from build123d import *

# Parameters (mm, degrees)
SKETCH1_R                                = 5
BOSS_EXTRUDE2_DEPTH                      = 115.57
CUT_EXTRUDE1_DEPTH                       = 2.54
TAP_DRILL_FOR_10_32_TAP1_D               = 4.0386
TAP_DRILL_FOR_10_32_TAP1_DEPTH           = 11.486682152
TAP_DRILL_FOR_10_32_TAP1_TIP             = 1.213317848
TAP_DRILL_FOR_10_32_TAP1_ON_FACE_2_D     = 4.0386
TAP_DRILL_FOR_10_32_TAP1_ON_FACE_2_DEPTH = 11.486682152
TAP_DRILL_FOR_10_32_TAP1_ON_FACE_2_TIP   = 1.213317848


with BuildPart() as part:
    # Sketch1 → Boss-Extrude2 (new body)
    with BuildSketch(Plane(origin=(0, 0, 0), x_dir=(1, 0, 0), z_dir=(0, 1, 0))):
        Circle(SKETCH1_R)
    extrude(amount=-BOSS_EXTRUDE2_DEPTH)

    # Sketch2 → Cut-Extrude1 (cut)
    with BuildSketch(Plane(origin=(0, 0, -5), x_dir=(-1, 0, 0), z_dir=(0, 0, -1))):
        with BuildLine():
            Line((-2, -109.22), (-2, -114.22))
            ThreePointArc((-2, -114.22), (0, -116.22), (2, -114.22))
            Line((2, -114.22), (2, -109.22))
            ThreePointArc((2, -109.22), (0, -107.22), (-2, -109.22))
        make_face()
        with BuildLine():
            Line((-1.5, -63.5), (-1.5, -68.5))
            ThreePointArc((-1.5, -68.5), (0, -70), (1.5, -68.5))
            Line((1.5, -68.5), (1.5, -63.5))
            ThreePointArc((1.5, -63.5), (0, -62), (-1.5, -63.5))
        make_face()
        with BuildLine():
            Line((-1.5, -10.39), (-1.5, -15.39))
            ThreePointArc((-1.5, -15.39), (0, -16.89), (1.5, -15.39))
            Line((1.5, -15.39), (1.5, -10.39))
            ThreePointArc((1.5, -10.39), (0, -8.89), (-1.5, -10.39))
        make_face()
    extrude(amount=-CUT_EXTRUDE1_DEPTH, mode=Mode.SUBTRACT)

    # Tap Drill for #10-32 Tap1
    with Locations(Plane.ZX):
        with Locations((0, 0)):
            Hole(TAP_DRILL_FOR_10_32_TAP1_D / 2, depth=TAP_DRILL_FOR_10_32_TAP1_DEPTH)
            with Locations((0, 0, -(TAP_DRILL_FOR_10_32_TAP1_DEPTH + TAP_DRILL_FOR_10_32_TAP1_TIP / 2))):  # 118° drill point
                Cone(0, TAP_DRILL_FOR_10_32_TAP1_D / 2, TAP_DRILL_FOR_10_32_TAP1_TIP, mode=Mode.SUBTRACT)

    # Tap Drill for #10-32 Tap1 on face 2
    with Locations(Plane(origin=(0, -115.57, 0), x_dir=(0, 0, -1), z_dir=(0, -1, 0))):
        with Locations((0, 0)):
            Hole(TAP_DRILL_FOR_10_32_TAP1_ON_FACE_2_D / 2, depth=TAP_DRILL_FOR_10_32_TAP1_ON_FACE_2_DEPTH)
            with Locations((0, 0, -(TAP_DRILL_FOR_10_32_TAP1_ON_FACE_2_DEPTH + TAP_DRILL_FOR_10_32_TAP1_ON_FACE_2_TIP / 2))):  # 118° drill point
                Cone(0, TAP_DRILL_FOR_10_32_TAP1_ON_FACE_2_D / 2, TAP_DRILL_FOR_10_32_TAP1_ON_FACE_2_TIP, mode=Mode.SUBTRACT)


solid = part.part
Geometry check sheet. Reference: the model listing, model coordinates, mm. A direction names the side the tool comes from. Give positions to 0.01 mm unless a question says otherwise; leave off trailing zeros. Loops run counter-clockwise (first coordinate to the right, second up) from the corner with the lowest first, then second, coordinate; pieces in that order, holes last. Notation, with made-up numbers: M 29.25,65 L 38.25,65 A26 cw 38.25,87 Z; hole C -9.75,-40 d11. An arc over 180 degrees is marked long. Answer as a JSON object with one key per item and string values. Group by question number.
Item 1: Sectioned sample at B-B on y = -90.5. Record the boundary of the cut face in (x, z).
Item 2: Gauge pin test, flat ends, axial feed: pin 1 (2.5 mm diameter, centred on x = 0.5, y = -14.5, fed in from -Z); pin 2 (1.2 mm diameter, centred on y = -66.5, z = -4, fed in from +X); pin 3 (3.5 mm diameter, centred on x = 0, z = 0, fed in from +Y). Record the tip position at first contact, or that the pin passes through.
Item 3: Material ranges on L1, parallel to X at y = -113, z = 0; L2, parallel to Z at x = 0, y = -107.75, recorded low to high.
Item 4: Access from +Z, -Z, +X, -X, +Y, -Y to the whole of each face (thin tool, end or side, straight path). Record for faces 1 (the cylindrical face through (0.03, -16.89, -3.75)), 2 (the cylindrical face through (0.607, -5.824, -1.926)), 3 (the cylindrical face through (-1.08, -56.98, 4.88)).
Item 5: Sectioned sample at A-A on z = 3. Record the boundary of the cut face in (x, y), plus the area to 3 significant figures.
Item 6: Mould release check, pull along Y, two halves, no side actions. Record for faces 4 (the cylindrical face through (-0.03, -8.89, -3.75)), 5 (the flat face through (-0.1, 0, 2.2)), 6 (the cylindrical face through (0.607, -109.746, 1.926)): pulls with the +Y half, pulls with the -Y half, needs draft (parallel to the pull), parting line crosses it, or undercut.
Findings below:
{
 "1": {"outline": "C 0,0 d10"},
 "2": {"pin 1": "z = -4.77", "pin 2": "x = 3.67", "pin 3": "y = -11.65"},
 "3": {"L1": "-5 to -2.02, 2.02 to 5", "L2": "-2.46 to -2.02, 2.02 to 5"},
 "4": {"face 1": "-Z", "face 2": "+Y", "face 3": "+Y, -Y"},
 "5": {"outline": "M -4,-115.57 L 4,-115.57 L 4,0 L -4,0 Z", "area": "925 mm2"},
 "6": {"face 4": "undercut", "face 5": "pulls with the +Y half", "face 6": "needs draft"}
}
